Geometry check sheet. Reference: the model listing, model coordinates, mm. A direction names the side the tool comes from. Round coordinates to 2 decimals unless told otherwise and drop trailing zeros. Write each loop counter-clockwise with the first axis right and the second up, starting at its lowest first coordinate (ties: lowest second). Pieces come first, ordered by that corner, then holes. Notation, with made-up numbers: (20, 57) - (75, 57) arc R24 ccw to (75, 86) - close; hole circle Ø4 at (-30.5, 83.25). An arc over 180 degrees is marked (long way). Return JSON: item names as keys, results as strings. Group by question number.
from build123d import *

# Parameters (mm, degrees)
SKETCH1_W           = 270
SKETCH1_H           = 300
BOSS_EXTRUDE1_DEPTH = 10
SKETCH2_W           = 75
SKETCH2_H           = 146.65
CUT_EXTRUDE1_DEPTH  = 9
CUT_EXTRUDE1_DRAFT  = -45


with BuildPart() as part:
    # Sketch1 → Boss-Extrude1 (new body)
    with BuildSketch(Plane.XY):
        Rectangle(SKETCH1_W, SKETCH1_H)
    extrude(amount=BOSS_EXTRUDE1_DEPTH)


with BuildPart() as cut_extrude1_tool:
    # Sketch2 → Cut-Extrude1 (with draft: the straight prism first)
    with BuildSketch(Plane.XY.offset(10)):
        with Locations((-28.39, -76.675)):
            Rectangle(SKETCH2_W, SKETCH2_H)
    extrude(amount=-CUT_EXTRUDE1_DEPTH)
    # Cut-Extrude1: the draft: its side faces are tilted about the plane it starts from
    cut_extrude1_sides = [cut_extrude1_tool.faces().sort_by_distance(p)[0] for p in [
        (-28.39, -150, 5.5),
        (9.11, -76.675, 5.5),
        (-28.39, -3.35, 5.5),
        (-65.89, -76.675, 5.5),
    ]]
    draft(cut_extrude1_sides, Plane.XY.offset(10), CUT_EXTRUDE1_DRAFT)


with BuildPart() as part_1:
    add(part.part)

    # Cut-Extrude1: cut by cut_extrude1_tool
    add(cut_extrude1_tool.part, mode=Mode.SUBTRACT)


solid = part_1.part
1. Section check A-A (z = 7.25). Enter the section's corners in (x, y).
2. Depth check by flat-ended pin: pin 1 Ø10 at (x, y) = (-7.5, -92) entering from +Z. Enter the tip coordinate at first touch or a pass-through.
3. Section check C-C (y = -99.5). Enter the section's corners in (x, z).
4. Tool access check on faces 4 (the face through (-2, 2, 10)), 5 (the face through (-28.92, -7.79, 5.56)). Record the directions out of +Z, -Z, +X, -X, +Y, -Y that give a thin tool (end or side, any length) a straight path to the whole face; none if there is none.
5. Material ranges on line 1 along X through (y, z) = (-103.5, 1.5); line 2 along X through (y, z) = (-28.5, 2.5); line 3 along Y through (x, z) = (-28.5, 8.5), recorded low to high.
6. Section check B-B (x = -34.5). Enter the section's corners in (y, z), and give its area (3 significant figures).
7. Mould release check, pull along Y, two halves, no side actions. Record for faces 1 (the face through (135, -2, 5)), 2 (the face through (-61.45, -77.7, 5.56)), 3 (the face through (-2, 150, 5)): pulls with the +Y half, pulls with the -Y half, needs draft (parallel to the pull), parting line crosses it, or undercut.
Result sheet:
{
 "1": {"outline": "(-135, -150) - (135, -150) - (135, 150) - (-135, 150) - close; hole (-63.14, -147.25) - (6.36, -147.25) - (6.36, -6.1) - (-63.14, -6.1) - close"},
 "2": {"pin 1": "stops at z = 1"},
 "3": {"outline": "(-135, 0) - (135, 0) - (135, 10) - (9.11, 10) - (0.11, 1) - (-56.89, 1) - (-65.89, 10) - (-135, 10) - close"},
 "4": {"face 4": "+Z, +X, -X, +Y, -Y", "face 5": "+Z"},
 "5": {"line 1": "x = -135 to -57.39, 0.61 to 135", "line 2": "x = -135 to -58.39, 1.61 to 135", "line 3": "y = -150 to -148.5, -4.85 to 150"},
 "6": {"outline": "(-150, 0) - (150, 0) - (150, 10) - (-3.35, 10) - (-12.35, 1) - (-141, 1) - (-150, 10) - close", "area": "1,760 mm²"},
 "7": {"face 1": "needs draft", "face 2": "undercut", "face 3": "pulls with the +Y half"}
}
